from build123d import *

# Parameters (mm, degrees)
SKETCH1_R           = 0.1
BOSS_EXTRUDE1_DEPTH = 0.18
FILLET1_R           = 0.5
FILLET2_R           = 0.7


# Some blends are built 0.0001 mm under size
with BuildPart() as part:
    # Sketch1 → Boss-Extrude1 (new body)
    with BuildSketch(Plane(origin=(0, 0, 0), x_dir=(1, 0, 0), z_dir=(0, 1, 0))):
        with BuildLine():
            Line((-0.5, -4.214213562), (-0.5, -1.414213562))
            ThreePointArc((-0.5, -1.414213562), (-1.5, 0), (-0.5, 1.414213562))
            Line((-0.5, 1.414213562), (-0.5, 10.785786438))
            Line((-0.5, 10.785786438), (0.5, 10.785786438))
            Line((0.5, 10.785786438), (0.5, 1.414213562))
            ThreePointArc((0.5, 1.414213562), (1.5, 0), (0.5, -1.414213562))
            Line((0.5, -1.414213562), (0.5, -4.214213562))
            Line((0.5, -4.214213562), (-0.5, -4.214213562))
        make_face()
        with Locations(Location((0, 0, 0), (0, 0, 270))):
            Circle(SKETCH1_R, mode=Mode.SUBTRACT)
    extrude(amount=BOSS_EXTRUDE1_DEPTH)

    # Fillet1
    fillet1_edges = [part.edges().sort_by_distance(p)[0] for p in [
        (-0.5, 0.09, 4.214213562),
        (0.5, 0.09, 4.214213562),
    ]]
    fillet(fillet1_edges, radius=FILLET1_R - 0.0001)  # a hair under: the kernel refuses the full size

    # Fillet2
    # the kernel refuses this fillet: 0.7 mm, written as the material it takes off along each edge
    with BuildSketch(Plane(origin=(-0.5, -1.75, -10.785786438), x_dir=(1, 0, 0), z_dir=(0, 1, 0)), Plane(origin=(0.5, -1.75, -10.785786438), x_dir=(0, 0, 1), z_dir=(0, 1, 0))) as fillet2_piece_1:
        with BuildLine():
            CenterArc((FILLET2_R, -FILLET2_R), FILLET2_R, 90, 90)
            Line((0, -FILLET2_R), (0, 0))
            Line((0, 0), (FILLET2_R, 0))
        make_face()
    extrude(amount=3.68, mode=Mode.SUBTRACT)


solid = part.part
CAD build for the part. Positions are in the model's coordinates, mm. Round coordinates to 2 decimals unless told otherwise and drop trailing zeros. Write each loop counter-clockwise with the first axis right and the second up, starting at its lowest first coordinate (ties: lowest second). Pieces come first, ordered by that corner, then holes. Notation, with made-up numbers: M 19,42 L 41,42 A21 cw 41,75 Z; hole C 32,54.5 d8. An arc over 180 degrees is marked long. Put each result on its own line as item: value. Start each with the question number.
1) Saw through at B-B, the plane z = -3.5. Write the cut outline in (x, y), and give its area (3 significant figures).
2) Drill centre lines: probe 1 along X at (y, z) = (0.1, 0); probe 2 along X at (y, z) = (0.1, -4.25); probe 3 along X at (y, z) = (0.1, 0.5). Where is each one in solid material? Low to high. Write a range as [from, to].
3) Saw through at C-C, the plane x = 0.95. Write the cut outline in (y, z).
Resolved:
1. outline: M -0.5,0 L 0.5,0 L 0.5,0.18 L -0.5,0.18 Z
1. area: 0.180 mm²
2. probe 1: [-1.5, -0.1], [0.1, 1.5]
2. probe 2: [-0.5, 0.5]
2. probe 3: [-1.41, 1.41]
3. outline: M 0,-1.16 L 0.18,-1.16 L 0.18,1.16 L 0,1.16 Z
